The model under review builds one solid part; all positions refer to its coordinate system, in mm. Face numbers are marked on the shaded views. Round coordinates to 2 decimals unless told otherwise and drop trailing zeros. Write each loop counter-clockwise with the first axis right and the second up, starting at its lowest first coordinate (ties: lowest second). Pieces come first, ordered by that corner, then holes. Notation, with made-up numbers: (53, 40.25) -> (64, 40.25) arc R30 cw to (64, 75.25) -> close; hole circle Ø5 at (62.5, 55). An arc over 180 degrees is marked (long way). Return JSON: item names as keys, results as strings. Group by question number.
1. For line 1 along Z through (x, y) = (-0.5, 4.5); line 2 along X through (y, z) = (1.25, 2.5); line 3 along Z through (x, y) = (1.75, 2), list the stretches that pass through material, from the lowest coordinate up. Write a range as from..to.
2. Mouldability with a two-part tool opening along X and no side actions: class the marked faces 1, 2, 3 and 4 as pulls with the +X half, pulls with the -X half, needs draft (parallel to the pull), parting line crosses it, or undercut.
3. Take a section at D-D, the plane y = 0.5. Give the number of separate pieces and of enclosed holes in the cut face, then the cut area to 3 significant figures.
4. Clearance check with a flat-ended pin moving along its axis: P1, Ø6, axis at x = -0.5, z = -0.5, coming from the -Y side. State where the tip first meets the part, or that it passes through.
5. Take a section at A-A, the plane z = -4.5. Write out the cut boundary in (x, y), then the cut area to 3 significant figures.
6. Take a section at C-C, the plane z = 0. Write out the cut boundary in (x, y).
7. Take a section at B-B, the plane x = 2. Write out the cut boundary in (y, z), then the cut area to 3 significant figures.
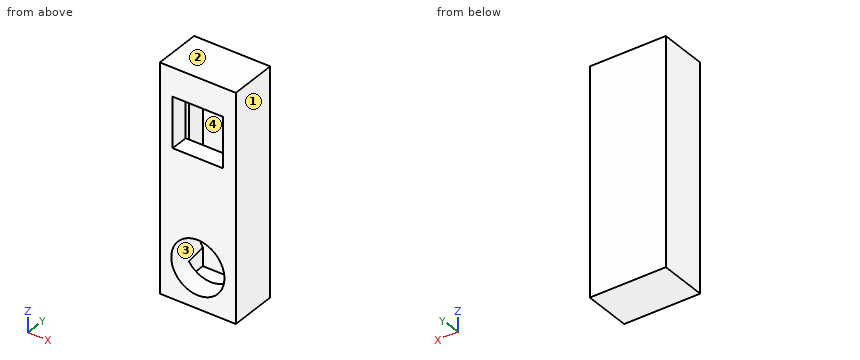
from build123d import *

# Parameters (mm, degrees)
SKETCH1_W           = 11.8
SKETCH1_H           = 35
SKETCH1_W_2         = 7.8
SKETCH1_H_2         = 7.8
BOSS_EXTRUDE1_DEPTH = 2.8
SKETCH2_W           = 11.8
SKETCH2_H           = 35
BOSS_EXTRUDE2_DEPTH = 3
SKETCH3_W           = 11.8
SKETCH3_H           = 35
BOSS_EXTRUDE3_DEPTH = 1.6
CUT_EXTRUDE1_REACH  = 15.365
SKETCH4_R           = 4.125


with BuildPart() as part:
    # Sketch1 → Boss-Extrude1 (new body)
    with BuildSketch(Plane(origin=(0, 0, 0), x_dir=(1, 0, 0), z_dir=(0, 1, 0))):
        with Locations((0, 9.2)):
            Rectangle(SKETCH1_W, SKETCH1_H)
        Rectangle(SKETCH1_W_2, SKETCH1_H_2, mode=Mode.SUBTRACT)
    extrude(amount=BOSS_EXTRUDE1_DEPTH)

    # Sketch2 → Boss-Extrude2 (add)
    with BuildSketch(Plane(origin=(0, 2.8, 0), x_dir=(1, 0, 0), z_dir=(0, 1, 0))):
        with Locations((0, 9.2)):
            Rectangle(SKETCH2_W, SKETCH2_H)
        Polygon((-3.9, 3.9), (-3.4, 3.9), (-3.4, 24.7), (3.4, 24.7), (3.4, 3.9), (3.9, 3.9), (3.9, -3.9), (-3.9, -3.9), align=None, mode=Mode.SUBTRACT)
        Polygon((3.4, -3.4), (-3.4, -3.4), (-3.4, 3.4), (-3.4, 3.9), (-3.9, 3.9), (-3.9, -3.9), (3.9, -3.9), (3.9, 3.9), (3.4, 3.9), (3.4, 3.4), align=None)
    extrude(amount=BOSS_EXTRUDE2_DEPTH)

    # Sketch3 → Boss-Extrude3 (add)
    with BuildSketch(Plane(origin=(0, 5.8, 0), x_dir=(1, 0, 0), z_dir=(0, 1, 0))):
        with Locations((0, 9.2)):
            Rectangle(SKETCH3_W, SKETCH3_H)
    extrude(amount=BOSS_EXTRUDE3_DEPTH)

    # Cut-Extrude1: up to this face of the body (flat: up to its plane)
    cut_extrude1_end = Plane(part.part.faces().sort_by_distance((0, 5.8, -10.65))[0])
    # Sketch4 → Cut-Extrude1 (cut, up to the picked face)
    with BuildSketch(Plane(origin=(0, -4.565968913, -0.805103513), x_dir=(-1, 0, 0), z_dir=(0, -0.984807753, -0.173648178)), mode=Mode.PRIVATE) as cut_extrude1_sk1:
        with Locations((0, 20.169367005)):
            Circle(SKETCH4_R)
    cut_extrude1_tool1 = split(extrude(cut_extrude1_sk1.sketch, amount=-CUT_EXTRUDE1_REACH, mode=Mode.PRIVATE), bisect_by=cut_extrude1_end, keep=Keep.BOTH, mode=Mode.PRIVATE)
    add(cut_extrude1_tool1.solids().sort_by_distance((0, -1.063595, -20.668053))[0], mode=Mode.SUBTRACT)


solid = part.part
Output:
{
 "1": {"line 1": "z = -26.7..-24.7, 3.4..8.3", "line 2": "x = -5.9..-3.9, 3.9..5.9", "line 3": "z = -26.7..-23.92, -16.33..-3.9, 3.9..8.3"},
 "2": {"face 1": "pulls with the +X half", "face 2": "needs draft", "face 3": "undercut", "face 4": "undercut"},
 "3": {"separate pieces": "1", "enclosed holes": "2", "area": "298 mm^2"},
 "4": {"P1": "stops at y = 2.8"},
 "5": {"outline": "(-5.9, 0) -> (5.9, 0) -> (5.9, 7.4) -> (-5.9, 7.4) -> close; hole (-3.4, 2.8) -> (3.4, 2.8) -> (3.4, 5.8) -> (-3.4, 5.8) -> close", "area": "66.9 mm^2"},
 "6": {"outline": "(-5.9, 0) -> (-3.9, 0) -> (-3.9, 2.8) -> (-3.4, 2.8) -> (-3.4, 5.8) -> (3.4, 5.8) -> (3.4, 2.8) -> (3.9, 2.8) -> (3.9, 0) -> (5.9, 0) -> (5.9, 7.4) -> (-5.9, 7.4) -> close"},
 "7": {"outline": "(0, -26.7) -> (7.4, -26.7) -> (7.4, 8.3) -> (0, 8.3) -> (0, 3.9) -> (2.8, 3.9) -> (2.8, 3.4) -> (5.8, 3.4) -> (5.8, -24.7) -> (2.8, -24.7) -> (2.8, -23.65) -> (0, -24.14) -> close; (0, -16.82) -> (2.8, -16.32) -> (2.8, -3.9) -> (0, -3.9) -> close", "area": "132 mm^2"}
}
